Could you check a few things on this model? Use its own coordinates, in mm. A direction names the side the tool comes from. Give positions to 0.01 mm unless a question says otherwise; leave off trailing zeros. Order: outer loops, then holes, each group sorted by start corner. A loop starts at its lowest first (then second) coordinate and runs counter-clockwise, first axis right, second up. Notation, with made-up numbers: (55, 33) -> (74, 33) arc R20 cw to (74, 51) -> close; hole circle Ø4 at (-10.75, 3.5). An arc over 180 degrees is marked (long way). One line per item, written item: value.
```python
from build123d import *

# Parameters (mm, degrees)
F4_DEPTH = 9.6
F5_R     = 1.483987


with BuildPart() as f1:
    # F0 (on Front) → F1 (revolve)
    with BuildSketch(Plane.XZ):
        Polygon((-5.8, 0), (0, 0), (0, 38.57), (-3, 38.57), (-3.916144, 31.5), (-3.916144, 4), (-5.8, 4), align=None)
    revolve(axis=Axis((0, 0, 19.285), (0, 0, -1)))

    # F3 (on offset) → F4 (cut)
    with BuildSketch(Plane.YZ.offset(3.215)):
        Polygon((-4.207731, 39.193626), (-4.207731, 4.065906), (4.512294, 4.065906), (4.867772, 39.193626), align=None)
    extrude(amount=F4_DEPTH, mode=Mode.SUBTRACT)

    # F5
    f5_edges = [f1.edges().sort_by_distance(p)[0] for p in [
        (3, 0, 38.57),
    ]]
    fillet(f5_edges, radius=F5_R)


solid = f1.part
```
1) Suppose I cut it at B-B, the plane x = 0. Write out the boundary of the cut face in (y, z).
Answer below:
outline: (-5.8, 0) -> (5.8, 0) -> (5.8, 4) -> (3.92, 4) -> (3.92, 31.5) -> (3.17, 37.28) arc R1.48 ccw to (1.7, 38.57) -> (-1.7, 38.57) arc R1.48 ccw to (-3.17, 37.28) -> (-3.92, 31.5) -> (-3.92, 4) -> (-5.8, 4) -> close
2) For faces 1 (the flat face through (1, -4, 4)), 2 (the cylindrical face through (5.794, 0.255, 1.972)), which set-ups out of +Z, -Z, +X, -X, +Y, -Y let a thin tool reach every point of the face, with its end or its side?
Answer below:
face 1: +Z
face 2: +Z, -Z
3) If I drill on line 1 along Z through (x, y) = (-3, -4); line 2 along Z through (x, y) = (3.25, 1); line 3 along X through (y, z) = (0.5, 31.5) (3 decimals), over which ranges is the centre line in solid material (lowest first)?
Answer below:
line 1: z = 0 to 4
line 2: z = 0 to 4.07
line 3: x = -3.884 to 3.215
4) Suppose I cut it at C-C, the plane z = 8. Write out the boundary of the cut face in (x, y) (3 decimals), then the cut area to 3 significant figures.
Answer below:
outline: (3.215, -2.236) -> (3.215, 2.236) arc R3.916 ccw (long way) to start
area: 46.0 mm2
5) Suppose I cut it at A-A, the plane y = 0. Write out the boundary of the cut face in (x, z) (3 decimals).
Answer below:
outline: (-5.8, 0) -> (5.8, 0) -> (5.8, 4) -> (3.916, 4) -> (3.916, 4.066) -> (3.215, 4.066) -> (3.215, 36.911) -> (3.168, 37.277) arc R1.484 ccw to (1.696, 38.57) -> (-1.696, 38.57) arc R1.484 ccw to (-3.168, 37.277) -> (-3.916, 31.5) -> (-3.916, 4) -> (-5.8, 4) -> close
6) For P1, Ø2, axis at y = 0.5, z = 13, coming from the +X side (3 decimals); P2, Ø6, axis at y = -2.5, z = 17, coming from the -X side; P3, Ø2, axis at x = 4.5, z = 31, coming from the +Y side; P4, Ø2, axis at x = 4, y = -2, coming from the -Z side, each with a flat end and sliding along its axis, tell me the tip position at first contact or that it passes through.
Answer below:
P1: stops at x = 3.215
P2: stops at x = -3.92
P3: passes through
P4: stops at z = 0
7) We'd pull the mould along X, two halves only. Please class faces 3 (the conical face through (-3.304, 1.04, 34.99)), 4 (the flat face through (3.215, 0, 21)), 5 (the flat face through (0, 0, 38.57)): +X half, -X half, draft (parallel to the pull), parting line (faces both ways), or undercut.
Answer below:
face 3: parting line
face 4: +X half
face 5: draft
8) Suppose I cut it at D-D, the plane z = 3. Write out the boundary of the cut face in (x, y).
Answer below:
outline: circle Ø11.6 at (0, 0)
